```python
from build123d import *

# Parameters (mm, degrees)
SKETCH_2_R      = 1.7
EXTRUDE_1_DEPTH = 5
SKETCH_9_W      = 12.5
SKETCH_9_H      = 5.5
EXTRUDE_5_DEPTH = 1
SKETCH_11_R     = 1.7
EXTRUDE_6_DEPTH = 3


with BuildPart() as part:
    # 草图2 → 凸台-拉伸1 (new body)
    with BuildSketch(Plane(origin=(0, 0, 0), x_dir=(1, 0, 0), z_dir=(0, 1, 0))):
        with Locations(Location((0, 0, 0), (0, 0, 270))):
            Circle(SKETCH_2_R)
    extrude(amount=-EXTRUDE_1_DEPTH)

    # 草图9 → 凸台-拉伸5 (add)
    with BuildSketch(Plane(origin=(0, 0, 0), x_dir=(1, 0, 0), z_dir=(0, 1, 0))):
        with Locations((1.75, 0)):
            Rectangle(SKETCH_9_W, SKETCH_9_H)
    extrude(amount=EXTRUDE_5_DEPTH)

    # 草图11 → 凸台-拉伸6 (add)
    with BuildSketch(Plane.XZ):
        with Locations(Location((5.3, 0, 0), (0, 0, 270))):
            Circle(SKETCH_11_R)
    extrude(amount=EXTRUDE_6_DEPTH)


solid = part.part
```
Check sheet for the modelled part. Datum: model origin and axes. Units: mm. A direction names the side the tool comes from. Round coordinates to 2 decimals unless told otherwise and drop trailing zeros. Order: outer loops, then holes, each group sorted by start corner. A loop starts at its lowest first (then second) coordinate and runs counter-clockwise, first axis right, second up. Notation, with made-up numbers: M -5.5,-39 L 6.5,-39 A26 ccw 6.5,0 Z; hole C 69.25,58 d7. An arc over 180 degrees is marked long. Answer in a Markdown table with one row per item.
(1) Section check D-D on x = 5.3. Record the boundary of the cut face in (y, z), plus the area to 3 significant figures.
Findings:
| item | result |
|---|---|
| outline | M -3,-1.7 L 0,-1.7 L 0,-2.75 L 1,-2.75 L 1,2.75 L 0,2.75 L 0,1.7 L -3,1.7 Z |
| area | 15.7 mm^2 |
(2) Section check C-C on y = -2.75. Record the boundary of the cut face in (x, z), plus the area to 3 significant figures.
Findings:
| item | result |
|---|---|
| outline | C 0,0 d3.4; C 5.3,0 d3.4 |
| area | 18.2 mm^2 |
(3) Section check A-A on z = 0. Record the boundary of the cut face in (x, y), plus the area to 3 significant figures.
Findings:
| item | result |
|---|---|
| outline | M -4.5,0 L -1.7,0 L -1.7,-5 L 1.7,-5 L 1.7,0 L 3.6,0 L 3.6,-3 L 7,-3 L 7,0 L 8,0 L 8,1 L -4.5,1 Z |
| area | 39.7 mm^2 |
(4) Material ranges on line 1 along Y through (x, z) = (3, -0.4); line 2 along Y through (x, z) = (6.5, -1.1); line 3 along X through (y, z) = (-1.4, -0.9), recorded low to high. Write a range as from..to.
Findings:
| item | result |
|---|---|
| line 1 | y = 0..1 |
| line 2 | y = -3..1 |
| line 3 | x = -1.44..1.44, 3.86..6.74 |
(5) Gauge pin test, flat ends, axial feed: pin 1 (1.5 mm diameter, centred on x = -1, y = -2, fed in from -Z); pin 2 (1 mm diameter, centred on x = 5.5, z = -0.5, fed in from -Y). Record the tip position at first contact, or that the pin passes through.
Findings:
| item | result |
|---|---|
| pin 1 | stops at z = -1.68 |
| pin 2 | stops at y = -3 |
(6) Set-up check for faces 4 (the flat face through (2, 0, -1)), 5 (the flat face through (5, -3, 0)), 6 (the flat face through (1.7, 0.5, 2.75)): record each of +Z, -Z, +X, -X, +Y, -Y from which the full face is reachable in a straight line by a thin tool's end or side.
Findings:
| item | result |
|---|---|
| face 4 | -Y |
| face 5 | +Z, -Z, +X, -Y |
| face 6 | +Z, +X, -X, +Y, -Y |
(7) Section check B-B on x = 0. Record the boundary of the cut face in (y, z), plus the area to 3 significant figures.
Findings:
| item | result |
|---|---|
| outline | M -5,-1.7 L 0,-1.7 L 0,-2.75 L 1,-2.75 L 1,2.75 L 0,2.75 L 0,1.7 L -5,1.7 Z |
| area | 22.5 mm^2 |
(8) Draft check along X on faces 1 (the flat face through (8, 0.5, 0)), 2 (the flat face through (0, -5, 0)), 3 (the cylindrical face through (6.45, -1.48, 1.25)). Enter one of: +X half, -X half, draft (parallel to the pull), parting line (faces both ways), or undercut.
Findings:
| item | result |
|---|---|
| face 1 | +X half |
| face 2 | draft |
| face 3 | undercut |
